from build123d import *


with BuildPart() as f1:
    # F0 (on Front) → F1 (revolve)
    with BuildSketch(Plane.XZ):
        with BuildLine():
            Line((-21.7, 18.917404), (-21.7, 4))
            Line((-21.7, 4), (21.7, 4))
            Line((21.7, 4), (21.7, 18.917404))
            Line((21.7, 18.917404), (15, 18.917404))
            Line((15, 18.917404), (11, 18.917404))
            Line((11, 18.917404), (11, 38.301961))
            ThreePointArc((11, 38.301961), (0, 33.5), (-11, 38.301961))
            Line((-11, 38.301961), (-11, 18.917404))
            Line((-11, 18.917404), (-15, 18.917404))
            Line((-15, 18.917404), (-21.7, 18.917404))
        make_face()
        with BuildLine():
            ThreePointArc((15, 48.5), (-5.477226, 62.46424), (-11, 38.301961))
            ThreePointArc((-11, 38.301961), (0, 33.5), (11, 38.301961))
            ThreePointArc((11, 38.301961), (13.96424, 43.022774), (15, 48.5))
        make_face()
    revolve(axis=Axis((0, 0, 0), (1, 0, 0)))


solid = f1.part
Build history of the part. All positions in model axes, mm. A direction names the side the tool comes from. Coordinates: 2 decimals unless noted, no trailing zeros. Order: outer loops, then holes, each group sorted by start corner. A loop starts at its lowest first (then second) coordinate and runs counter-clockwise, first axis right, second up. Notation, with made-up numbers: (63.5, -18.75) - (72.5, -18.75) arc R23 cw to (72.5, -4.75) - close; hole circle Ø4 at (-5.5, -1). An arc over 180 degrees is marked (long way). Write item = value, one per line. Start each with the question number.
1) 3-axis set-ups, long thin cutter, end or side, ignore diameter. For faces 1 (the face through (11, 8, 18)), 2 (the face through (-16.425, 11.511, -15.012)), 3 (the face through (0.304, 3.905, -0.867)): which of +Z, -Z, +X, -X, +Y, -Y reach the whole face in a straight line?
2) Flat gauge pins, fed straight in: pin 1 Ø1.5 at (x, z) = (1.5, 38.5) entering from +Y; pin 2 Ø8 at (y, z) = (8, 44) entering from +X; pin 3 Ø1 at (y, z) = (25.5, 21) entering from +X. Where does each tip first touch, or does it go through?
3) Saw through at D-D on x = 1. Write the cut outline in (y, z).
4) Saw through at C-C on x = 19.5. Write the cut outline in (y, z), then the cut area to 3 significant figures.
5) Saw through at A-A on z = 0. Write the cut outline in (x, y).
6) Two-plate mould, pull along Y, no slides. Class faces 4 (the face through (-21.7, -4.5, -0.3)), 5 (the face through (-11, 8, -18)): pulls with the +Y half, pulls with the -Y half, needs draft (parallel to the pull), parting line crosses it, or undercut.
7) Wall check: line 1 along Y through (x, z) = (-12, -7.5); line 2 along Z through (x, y) = (12.5, -6.5); line 3 along X through (y, z) = (7, -32.5). Give the ranges that are in metal, low to high. Write a range as from..to.
From the geometry:
q1.face_1 = +X
q1.face_2 = -X
q1.face_3 = +X, -X
q2.pin_1 = 50.97
q2.pin_2 = 15
q2.pin_3 = 11
q3.outline = circle Ø126.93 at (0, 0); hole circle Ø8 at (0, 0)
q4.outline = circle Ø37.83 at (0, 0); hole circle Ø8 at (0, 0)
q4.area = 1,070 mm^2
q5.outline = (-21.7, -18.92) - (-11, -18.92) - (-11, -38.3) arc R15 ccw (long way) to (15, -48.5) arc R15 ccw to (11, -38.3) - (11, -18.92) - (21.7, -18.92) - (21.7, -4) - (-21.7, -4) - close; (-21.7, 4) - (21.7, 4) - (21.7, 18.92) - (11, 18.92) - (11, 38.3) arc R15 ccw to (15, 48.5) arc R15 ccw (long way) to (-11, 38.3) - (-11, 18.92) - (-21.7, 18.92) - close
q6.face_4 = needs draft
q6.face_5 = undercut
q7.line_1 = -57.01..-38.78, -17.37..17.37, 38.78..57.01
q7.line_2 = -56.42..-39.68, -17.77..17.77, 39.68..56.42
q7.line_3 = -11..11
